```python
from build123d import *

# Parameters (mm, degrees)
SKETCH1_W           = 2.54
SKETCH1_H           = 2.54
BOSS_EXTRUDE1_DEPTH = 20.32
FILLET1_R           = 1.27
SKETCH2_R           = 0.762
CUT_EXTRUDE1_DEPTH  = 21.635057548


with BuildPart() as part:
    # Sketch1 → Boss-Extrude1 (new body)
    with BuildSketch(Plane.XY):
        with Locations((-1.27, 1.27)):
            Rectangle(SKETCH1_W, SKETCH1_H)
    extrude(amount=BOSS_EXTRUDE1_DEPTH)

    # Fillet1
    fillet1_edges = [part.edges().sort_by_distance(p)[0] for p in [
        (-1.27, 0, 20.32),
        (-1.27, 2.54, 20.32),
    ]]
    fillet(fillet1_edges, radius=FILLET1_R - 0.0001)  # a hair under: the kernel refuses the full size

    # Sketch2 → Cut-Extrude1 (cut, through all)
    with BuildSketch(Plane(origin=(0, 0, 0), x_dir=(0, 0, -1), z_dir=(1, 0, 0))):
        with Locations(Location((-19.05, 1.27, 0), (0, 0, 90))):
            Circle(SKETCH2_R)
    extrude(amount=-CUT_EXTRUDE1_DEPTH, mode=Mode.SUBTRACT)


solid = part.part
```
Work out the finished part from the listing and answer in its coordinate system (mm). Give positions to 0.01 mm unless a question says otherwise; leave off trailing zeros. Loops run counter-clockwise (first coordinate to the right, second up) from the corner with the lowest first, then second, coordinate; pieces in that order, holes last. Notation, with made-up numbers: (-39, -0.75) -> (-7, -0.75) arc R16 cw to (-7, 30.25) -> close; hole circle Ø8 at (-39.75, -18). An arc over 180 degrees is marked (long way). Put each result on its own line as item: value. Start each with the question number.
Item 1: The part is cut by section D-D (y = 0.2). Give the vertices of the cut face in (x, z).
Item 2: The mould has two halves that part along Y. Classify faces 1 (the face through (-1, 2.54, 9)), 2 (the face through (-2.54, 1, 10)), 3 (the face through (-1.25, 1.68, 19.69)), 4 (the face through (-1.252, 0.362, 19.938)): released by +Y, released by -Y, zero draft, split by the parting line, or undercut.
Item 3: The part is cut by section C-C (y = 2.3). Give the vertices of the cut face in (x, z).
Item 4: Find the intervals of material crossed by L1, parallel to Z at x = -0.15, y = 1.3; L2, parallel to Z at x = -0.15, y = 1.7; L3, parallel to Z at x = -1.6, y = 2.2, in increasing order. Write a range as [from, to].
Item 5: The part is cut by section B-B (y = 1.45). Give the vertices of the cut face in (x, z), then the cut area to 3 significant figures.
Answers below:
1. outline: (-2.54, 0) -> (0, 0) -> (0, 19.73) -> (-2.54, 19.73) -> close
2. face 1: released by +Y
2. face 2: zero draft
2. face 3: undercut
2. face 4: released by -Y
3. outline: (-2.54, 0) -> (0, 0) -> (0, 19.79) -> (-2.54, 19.79) -> close
4. L1: [0, 18.29], [19.81, 20.32]
4. L2: [0, 18.42], [19.68, 20.25]
4. L3: [0, 19.91]
5. outline: (-2.54, 0) -> (0, 0) -> (0, 18.31) -> (-2.54, 18.31) -> close; (-2.54, 19.79) -> (0, 19.79) -> (0, 20.31) -> (-2.54, 20.31) -> close
5. area: 47.8 mm2
